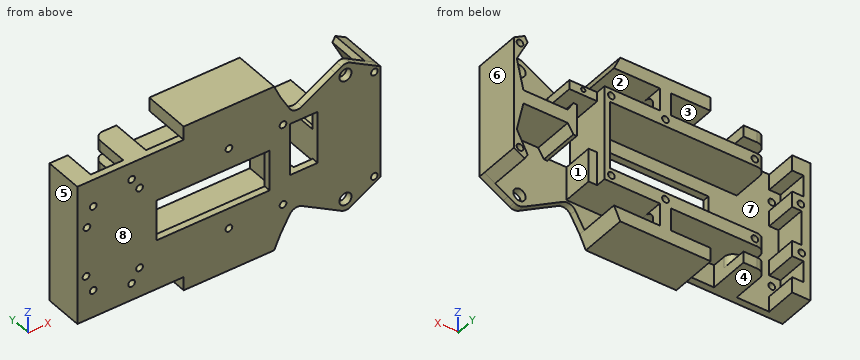
```python
from build123d import *

# Parameters (mm, degrees)
SKETCH_1_W               = 134
SKETCH_1_H               = 62
EXTRUDE_1_DEPTH          = 3
SKETCH_2_R               = 2.7
CUT_EXTRUDE_1_DEPTH      = 4
EXTRUDE_3_DEPTH          = 3
CUT_EXTRUDE_4_DEPTH      = 4
CUT_EXTRUDE_4_DEPTH_BACK = 3
SKETCH_1_6_W             = 12.3
SKETCH_1_6_H             = 23.1
SKETCH_3_W               = 4
SKETCH_3_H               = 15.4
EXTRUDE_4_DEPTH          = 14
SKETCH_4_W               = 5
SKETCH_4_H               = 5
EXTRUDE_5_DEPTH          = 18
FILLET_1_R               = 4
EXTRUDE_6_DEPTH          = 18
SKETCH_6_W               = 12.3
SKETCH_6_H               = 4.05
SKETCH_6_W_2             = 3.8
SKETCH_6_H_2             = 14.85
EXTRUDE_7_DEPTH          = 13.5
SKETCH_7_R               = 1.48
CUT_EXTRUDE_5_DEPTH      = 5
EXTRUDE_9_DEPTH          = 18
EXTRUDE_10_DEPTH         = 18
EXTRUDE_START            = -21
SKETCH_11_W              = 5
SKETCH_11_H              = 10
EXTRUDE_11_DEPTH         = 21
SKETCH_12_R              = 5
CUT_EXTRUDE_6_DEPTH      = 6
SKETCH_13_R              = 5
CUT_EXTRUDE_7_DEPTH      = 6
SKETCH_14_R              = 0.965
CUT_EXTRUDE_8_DEPTH      = 10
SKETCH_17_R              = 1.48
CUT_EXTRUDE_10_DEPTH     = 30
SKETCH_18_R              = 1.48
CUT_EXTRUDE_11_DEPTH     = 30
SKETCH_19_R              = 1.48
CUT_EXTRUDE_12_DEPTH     = 30
SKETCH_20_W              = 5
SKETCH_20_H              = 5
CUT_EXTRUDE_13_DEPTH     = 8
SKETCH_21_R              = 1.48
CUT_EXTRUDE_14_DEPTH     = 30
SKETCH_22_R              = 1.48
CUT_EXTRUDE_15_DEPTH     = 30
SKETCH_23_R              = 1.48
CUT_EXTRUDE_16_DEPTH     = 30
SKETCH_24_W              = 50
SKETCH_24_H              = 18
CUT_EXTRUDE_17_DEPTH     = 30
FILLET_2_R               = 4
FILLET_3_R               = 4


with BuildPart() as part:
    # 草图1 → 凸台-拉伸1 (new body)
    with BuildSketch(Plane(origin=(0, 0, 0), x_dir=(1, 0, 0), z_dir=(0, 1, 0))):
        Rectangle(SKETCH_1_W, SKETCH_1_H)
    extrude(amount=EXTRUDE_1_DEPTH)

    # 草图2 → 切除-拉伸1 (cut)
    with BuildSketch(Plane(origin=(0, 3, 0), x_dir=(1, 0, 0), z_dir=(0, 1, 0))):
        with Locations(Location((51.5, 28, 0), (0, 0, 270))):
            Circle(SKETCH_2_R)
        with Locations(Location((51.5, -28, 0), (0, 0, 270))):
            Circle(SKETCH_2_R)
    extrude(amount=-CUT_EXTRUDE_1_DEPTH, mode=Mode.SUBTRACT)

    # 草图1<4> → 凸台-拉伸3 (add)
    with BuildSketch(Plane(origin=(0, 0, 0), x_dir=(1, 0, 0), z_dir=(0, 1, 0))):
        Polygon((51.75, 33.742413779), (47, 31), (56.5, 31), align=None)
        Polygon((56.5, -31), (47, -31), (51.75, -33.742413779), align=None)
    extrude(amount=EXTRUDE_3_DEPTH)

    # 草图1<6> → 切除-拉伸4 (cut, two sides: drawn at the far end of the back side and taken through both)
    with BuildSketch(Plane(origin=(0, 0, 0), x_dir=(1, 0, 0), z_dir=(0, 1, 0)).offset(-CUT_EXTRUDE_4_DEPTH_BACK)):
        with Locations((33.065250205, -5.4)):
            Rectangle(SKETCH_1_6_W, SKETCH_1_6_H)
        Polygon((47, 31), (22.751288694, 31), (28.813466521, 20.5), align=None)
        Polygon((67, 31), (56.5, 31), (67, 24.937822174), align=None)
        Polygon((28.813466521, -20.5), (22.751288694, -31), (47, -31), align=None)
        Polygon((67, -24.937822174), (56.5, -31), (67, -31), align=None)
    extrude(amount=CUT_EXTRUDE_4_DEPTH + CUT_EXTRUDE_4_DEPTH_BACK, mode=Mode.SUBTRACT)

    # 草图3 → 凸台-拉伸4 (add)
    with BuildSketch(Plane(origin=(0, 3, 0), x_dir=(1, 0, 0), z_dir=(0, 1, 0))):
        Polygon((-58.9, 31), (-67, 31), (-67, 7.7), (-63, 7.7), (-58.9, 7.7), (-58.9, 14.6), (-63.9, 14.6), (-63.9, 24.1), (-58.9, 24.1), align=None)
        Polygon((-63, -7.7), (-67, -7.7), (-67, -31), (-58.9, -31), (-58.9, -24.1), (-63.9, -24.1), (-63.9, -14.6), (-58.9, -14.6), (-58.9, -7.7), align=None)
        with Locations((-65, 0)):
            Rectangle(SKETCH_3_W, SKETCH_3_H)
    extrude(amount=EXTRUDE_4_DEPTH)

    # 草图4 → 凸台-拉伸5 (add)
    with BuildSketch(Plane(origin=(0, 3, 0), x_dir=(1, 0, 0), z_dir=(0, 1, 0))):
        Polygon((24.5, 15), (24.5, 0), (26.915250205, 0), (26.915250205, 21), (24.5, 21), align=None)
        Polygon((26.915250205, 0), (24.5, 0), (24.5, -15), (24.5, -21), (26.915250205, -21), align=None)
        Polygon((-44.5, 15), (24.5, 15), (24.5, 21), (-34.5, 21), (-39.5, 21), (-44.5, 21), align=None)
        Polygon((24.5, -21), (24.5, -15), (-44.5, -15), (-44.5, -21), (-39.5, -21), (-34.5, -21), align=None)
        with Locations((-37, 23.5)):
            Rectangle(SKETCH_4_W, SKETCH_4_H)
        with Locations((-37, -23.5)):
            Rectangle(SKETCH_4_W, SKETCH_4_H)
        Polygon((-39.5, 26), (-34.5, 26), (-34.5, 31), (-44.5, 31), (-44.5, 26), align=None)
        Polygon((-34.5, -31), (-34.5, -26), (-39.5, -26), (-44.5, -26), (-44.5, -31), align=None)
    extrude(amount=EXTRUDE_5_DEPTH)

    # 圆角1
    fillet_1_edges = [part.edges().sort_by_distance(p)[0] for p in [
        (51.75, 1.5, 33.742413779),
        (28.813466521, 1.5, 20.5),
        (28.813466521, 1.5, -20.5),
        (51.75, 1.5, -33.742413779),
    ]]
    fillet(fillet_1_edges, radius=FILLET_1_R)

    # 草图5 → 凸台-拉伸6 (add)
    with BuildSketch(Plane(origin=(0, 3, 0), x_dir=(1, 0, 0), z_dir=(0, 1, 0))):
        Polygon((43.215250205, 3), (39.215250205, 3), (39.215250205, -3), (43.215250205, -3), (67, -3), (67, 3), align=None)
        Polygon((39.215250205, 6.15), (39.215250205, 3), (43.215250205, 3), (40.715250205, 7.102951113), (39.215250205, 7.102951113), align=None)
        Polygon((43.215250205, -3), (39.215250205, -3), (39.215250205, -7.102951113), (40.715250205, -7.102951113), align=None)
    extrude(amount=EXTRUDE_6_DEPTH)

    # 草图6 → 凸台-拉伸7 (add)
    with BuildSketch(Plane(origin=(0, 3, 0), x_dir=(1, 0, 0), z_dir=(0, 1, 0))):
        with Locations((33.065250205, -18.975)):
            Rectangle(SKETCH_6_W, SKETCH_6_H)
        with Locations((28.815250205, 13.575)):
            Rectangle(SKETCH_6_W_2, SKETCH_6_H_2)
    extrude(amount=EXTRUDE_7_DEPTH)

    # 草图7 → 切除-拉伸5 (cut)
    with BuildSketch(Plane.XZ):
        with Locations(Location((-60, 19, 0), (0, 0, 270))):
            Circle(SKETCH_7_R)
        with Locations(Location((-43, 23.5, 0), (0, 0, 270))):
            Circle(SKETCH_7_R)
        with Locations(Location((-43, -23.5, 0), (0, 0, 90))):
            Circle(SKETCH_7_R)
        with Locations(Location((-60, -19, 0), (0, 0, 90))):
            Circle(SKETCH_7_R)
    extrude(amount=-CUT_EXTRUDE_5_DEPTH, mode=Mode.SUBTRACT)

    # 草图9 → 凸台-拉伸9 (add)
    with BuildSketch(Plane(origin=(0, 3, 0), x_dir=(1, 0, 0), z_dir=(0, 1, 0))):
        Polygon((67, 3), (67, 24.937822174), (62.236860279, 27.687822174), (60.906181585, 25.383019067), (65.7, 15.937822174), (62.8, 3), align=None)
    extrude(amount=EXTRUDE_9_DEPTH)

    # 草图10 → 凸台-拉伸10 (add)
    with BuildSketch(Plane(origin=(0, 3, 0), x_dir=(1, 0, 0), z_dir=(0, 1, 0))):
        Polygon((67, -3), (62.8, -3), (65.7, -15.937822174), (60.906181585, -25.383019067), (62.236860279, -27.687822174), (67, -24.937822174), align=None)
    extrude(amount=EXTRUDE_10_DEPTH)

    # 草图11 → 凸台-拉伸11 (add)
    with BuildSketch(Plane.XZ.offset(EXTRUDE_START)):
        Polygon((-2.5, -31), (-20, -31), (-20, -37), (20, -37), (20, -31), (2.5, -31), align=None)
        with Locations((0, -26)):
            Rectangle(SKETCH_11_W, SKETCH_11_H)
        Polygon((20, -31), (20, -37), (22.751288694, -31), align=None)
        Polygon((2.5, 31), (20, 31), (20, 37), (-20, 37), (-20, 31), (-2.5, 31), align=None)
        with Locations((0, 26)):
            Rectangle(SKETCH_11_W, SKETCH_11_H)
        Polygon((20, 31), (22.751288694, 31), (20, 37), align=None)
    extrude(amount=EXTRUDE_11_DEPTH)

    # 草图12 → 切除-拉伸6 (cut)
    with BuildSketch(Plane.ZY.offset(2.5)):
        with Locations((26, 12)):
            Circle(SKETCH_12_R)
    extrude(amount=-CUT_EXTRUDE_6_DEPTH, mode=Mode.SUBTRACT)

    # 草图13 → 切除-拉伸7 (cut)
    with BuildSketch(Plane.ZY.offset(2.5)):
        with Locations((-26, 12)):
            Circle(SKETCH_13_R)
    extrude(amount=-CUT_EXTRUDE_7_DEPTH, mode=Mode.SUBTRACT)

    # 草图14 → 切除-拉伸8 (cut)
    with BuildSketch(Plane(origin=(0, 16.5, 0), x_dir=(1, 0, 0), z_dir=(0, 1, 0))):
        with Locations(Location((33.065250205, -19.325, 0), (0, 0, 270))):
            Circle(SKETCH_14_R)
    extrude(amount=-CUT_EXTRUDE_8_DEPTH, mode=Mode.SUBTRACT)

    # 草图17 → 切除-拉伸10 (cut)
    with BuildSketch(Plane(origin=(0, 21, 0), x_dir=(1, 0, 0), z_dir=(0, 1, 0))):
        with Locations(Location((64.3, 23.55, 0), (0, 0, 270))):
            Circle(SKETCH_17_R)
        with Locations(Location((64.3, -23.55, 0), (0, 0, 270))):
            Circle(SKETCH_17_R)
    extrude(amount=-CUT_EXTRUDE_10_DEPTH, mode=Mode.SUBTRACT)

    # 草图18 → 切除-拉伸11 (cut)
    with BuildSketch(Plane(origin=(0, 21, 0), x_dir=(1, 0, 0), z_dir=(0, 1, 0))):
        with Locations(Location((23.915250205, 18, 0), (0, 0, 270))):
            Circle(SKETCH_18_R)
        with Locations(Location((23.915250205, -18, 0), (0, 0, 270))):
            Circle(SKETCH_18_R)
    extrude(amount=-CUT_EXTRUDE_11_DEPTH, mode=Mode.SUBTRACT)

    # 草图19 → 切除-拉伸12 (cut)
    with BuildSketch(Plane(origin=(0, 21, 0), x_dir=(1, 0, 0), z_dir=(0, 1, 0))):
        with Locations(Location((0, 18, 0), (0, 0, 270))):
            Circle(SKETCH_19_R)
        with Locations(Location((0, -18.075939793, 0), (0, 0, 270))):
            Circle(SKETCH_19_R)
    extrude(amount=-CUT_EXTRUDE_12_DEPTH, mode=Mode.SUBTRACT)

    # 草图20 → 切除-拉伸13 (cut)
    with BuildSketch(Plane(origin=(0, 21, 0), x_dir=(1, 0, 0), z_dir=(0, 1, 0))):
        with Locations((-37, 23.5)):
            Rectangle(SKETCH_20_W, SKETCH_20_H)
        with Locations((-37, -23.5)):
            Rectangle(SKETCH_20_W, SKETCH_20_H)
    extrude(amount=-CUT_EXTRUDE_13_DEPTH, mode=Mode.SUBTRACT)

    # 草图21 → 切除-拉伸14 (cut)
    with BuildSketch(Plane(origin=(0, 21, 0), x_dir=(1, 0, 0), z_dir=(0, 1, 0))):
        with Locations(Location((-39.5, 18, 0), (0, 0, 270))):
            Circle(SKETCH_21_R)
        with Locations(Location((-39.5, -18, 0), (0, 0, 270))):
            Circle(SKETCH_21_R)
    extrude(amount=-CUT_EXTRUDE_14_DEPTH, mode=Mode.SUBTRACT)

    # 草图22 → 切除-拉伸15 (cut)
    with BuildSketch(Plane(origin=(0, 17, 0), x_dir=(1, 0, 0), z_dir=(0, 1, 0))):
        with Locations(Location((-63.15, 11.2, 0), (0, 0, 270))):
            Circle(SKETCH_22_R)
    extrude(amount=-CUT_EXTRUDE_15_DEPTH, mode=Mode.SUBTRACT)

    # 草图23 → 切除-拉伸16 (cut)
    with BuildSketch(Plane(origin=(0, 17, 0), x_dir=(1, 0, 0), z_dir=(0, 1, 0))):
        with Locations(Location((-62.75, -10.701666204, 0), (0, 0, 270))):
            Circle(SKETCH_23_R)
    extrude(amount=-CUT_EXTRUDE_16_DEPTH, mode=Mode.SUBTRACT)

    # 草图24 → 切除-拉伸17 (cut)
    with BuildSketch(Plane(origin=(0, 3, 0), x_dir=(1, 0, 0), z_dir=(0, 1, 0))):
        with Locations((-7, 0)):
            Rectangle(SKETCH_24_W, SKETCH_24_H)
    extrude(amount=-CUT_EXTRUDE_17_DEPTH, mode=Mode.SUBTRACT)

    # 圆角2
    # the kernel refuses this fillet: 4 mm, written as the material it takes off along each edge
    with BuildSketch(Plane(origin=(-44.5, 21, 5), x_dir=(1, 0, 0), z_dir=(0, 0, 1)), Plane(origin=(-44.5, 21, -31), x_dir=(1, 0, 0), z_dir=(0, 0, 1))) as fillet_2_piece_1:
        with BuildLine():
            CenterArc((FILLET_2_R, -FILLET_2_R), FILLET_2_R, 90, 90)
            Line((0, -FILLET_2_R), (0, 0))
            Line((0, 0), (FILLET_2_R, 0))
        make_face()
    extrude(amount=26, mode=Mode.SUBTRACT)
    with BuildSketch(Plane(origin=(-44.5, 21, -41), x_dir=(1, 0, 0), z_dir=(0, 0, 1))) as fillet_2_piece_2:
        with BuildLine():
            CenterArc((FILLET_2_R, -FILLET_2_R), FILLET_2_R, 90, 90)
            Line((0, -FILLET_2_R), (0, 0))
            Line((0, 0), (FILLET_2_R, 0))
        make_face()
    extrude(amount=25, mode=Mode.SUBTRACT)
    with BuildSketch(Plane(origin=(-44.5, 21, 16), x_dir=(0, -1, 0), z_dir=(0, 0, 1))) as fillet_2_piece_3:
        with BuildLine():
            CenterArc((FILLET_2_R, FILLET_2_R), FILLET_2_R, 180, 90)
            Line((0, FILLET_2_R), (0, 0))
            Line((0, 0), (FILLET_2_R, 0))
        make_face()
    extrude(amount=25, mode=Mode.SUBTRACT)

    # 圆角3
    fillet_3_edges = [part.edges().sort_by_distance(p)[0] for p in [
        (-34.5, 13, -23.5),
        (-34.5, 13, 23.5),
    ]]
    fillet(fillet_3_edges, radius=FILLET_3_R)


solid = part.part
```
CAD build for the part. Positions are in the model's coordinates, mm. Face numbers are marked on the shaded views. A direction names the side the tool comes from. Coordinates: 2 decimals unless noted, no trailing zeros. Loops run counter-clockwise (first coordinate to the right, second up) from the corner with the lowest first, then second, coordinate; pieces in that order, holes last. Notation, with made-up numbers: (82, 47) - (136, 47) arc R11 ccw to (136, 59) - close; hole circle Ø8 at (73, 20.25). An arc over 180 degrees is marked (long way). Use CSV: the item, a comma, the result in double quotes. Start each with the question number.
Q1. Cut at A-A, the plane z = -29. List the corners of the cut face in (x, y).
Q2. 3-axis set-ups, long thin cutter, end or side, ignore diameter. For the marked faces 1, 2, 3 and 4: which of +Z, -Z, +X, -X, +Y, -Y reach the whole face in a straight line?
Q3. Cut at B-B, the plane x = 64.3. List the corners of the cut face in (y, z).
Q4. Probe probe 1 along Z at (x, y) = (7, 18.25); probe 2 along Z at (x, y) = (24, 6.5); probe 3 along Z at (x, y) = (-25.5, 10). List the from-to ranges inside material, lowest first. Write a range as from..to.
Q5. Drop flat-ended pins along their axis: P1, Ø2, axis at x = 32, z = 18.5, coming from the +Y side; P2, Ø5, axis at x = -10.5, z = -18, coming from the -Y side; P3, Ø8, axis at x = -32, y = 4, coming from the +Z side; P4, Ø0.6, axis at x = 33.5, z = 19, coming from the +Y side. Give the stop position or say it passes through.
Q6. Two-plate mould, pull along X, no slides. Class the marked faces 5, 6, 7 and 8: +X half, -X half, draft (parallel to the pull), parting line (faces both ways), or undercut.
Q7. Cut at C-C, the plane y = 15.25. State how many separate pieces and enclosed holes the cut face has, then the cut area to 3 significant figures.
Here are the results:
1,outline,"(-67, 0) - (23.91, 0) - (23.91, 3) - (2.5, 3) - (2.5, 8) - (-2.5, 8) - (-2.5, 3) - (-34.5, 3) - (-34.5, 21) - (-40.5, 21) arc R4 ccw to (-44.5, 17) - (-44.5, 3) - (-58.9, 3) - (-58.9, 17) - (-67, 17) - close; (-2.5, 16) - (2.5, 16) - (2.5, 21) - (-2.5, 21) - close; (43.54, 0) - (48.99, 0) - (48.99, 3) - (43.54, 3) - close; (54.01, 0) - (59.96, 0) - (59.96, 3) - (54.01, 3) - close"
2,face 1,"-Z, +Y"
2,face 2,"+X, +Y"
2,face 3,"+Y"
2,face 4,"-Z, -X, +Y, -Y"
3,outline,"(0, -26.5) - (21, -26.5) - (21, -25.03) - (0, -25.03) - close; (0, -22.07) - (21, -22.07) - (21, -18.7) - (3, -18.7) - (3, -9.69) - (21, -9.69) - (21, 9.69) - (3, 9.69) - (3, 18.7) - (21, 18.7) - (21, 22.07) - (0, 22.07) - close; (0, 25.03) - (21, 25.03) - (21, 26.5) - (0, 26.5) - close"
4,probe 1,"-37..-31, -21..-15, 15..21, 31..37"
4,probe 2,"-21..-19.48, -16.52..-15, 15..16.52, 19.48..21"
4,probe 3,"-21..-15, 15..21"
5,P1,"y = 16.5"
5,P2,"y = 0"
5,P3,"z = 31"
5,P4,"y = 6.5"
6,face 5,"-X half"
6,face 6,"+X half"
6,face 7,"undercut"
6,face 8,"draft"
7,separate pieces,"7"
7,enclosed holes,"11"
7,area,"2,270 mm2"
